Part model, mm, in its own coordinate system. Face numbers are marked on the shaded views. Round coordinates to 2 decimals unless told otherwise and drop trailing zeros. Loops run counter-clockwise (first coordinate to the right, second up) from the corner with the lowest first, then second, coordinate; pieces in that order, holes last.
from build123d import *

# Parameters (mm, degrees)
SKETCH1_W                   = 135
SKETCH1_H                   = 25
BOSS_EXTRUDE1_DEPTH         = 6
TAP_DRILL_FOR_M6X1_0_TAP1_D = 5
SKETCH2_R                   = 8
CUT_EXTRUDE1_DEPTH          = 70.688593041


with BuildPart() as part:
    # Sketch1 → Boss-Extrude1 (new, symmetric)
    with BuildSketch(Plane.XY):
        Rectangle(SKETCH1_W, SKETCH1_H)
    extrude(amount=BOSS_EXTRUDE1_DEPTH, both=True)

    # Tap Drill for M6x1.0 Tap1 (through all)
    with Locations(Plane.XY.offset(6)):
        with Locations((-22.5, 6), (-22.5, -6), (22.5, 6), (22.5, -6)):
            Hole(TAP_DRILL_FOR_M6X1_0_TAP1_D / 2)

    # Sketch2 → Cut-Extrude1 (cut, through all)
    with BuildSketch(Plane.XY.offset(6)):
        with Locations((-57.7, 0)):
            Circle(SKETCH2_R)
        with Locations((57.7, 0)):
            Circle(SKETCH2_R)
    extrude(amount=-CUT_EXTRUDE1_DEPTH, mode=Mode.SUBTRACT)


solid = part.part
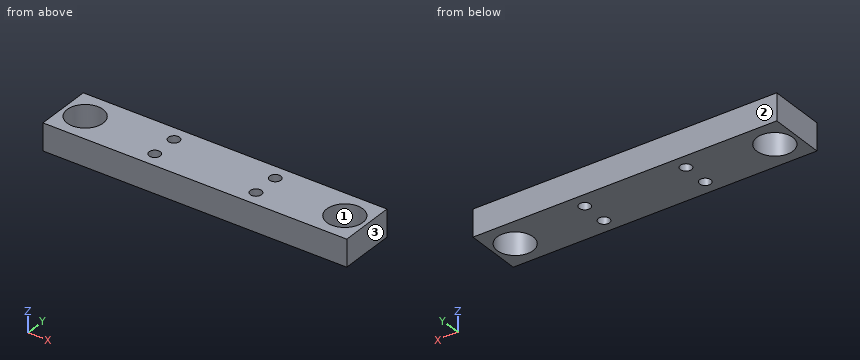
1) Wall check: line 1 along Y through (x, z) = (-22.5, 0); line 2 along X through (y, z) = (-0.5, -4.5); line 3 along Y through (x, z) = (-57.7, -0.5). Give the ranges that are in metal, low to high.
Values:
line 1: y = -12.5 to -8.5, -3.5 to 3.5, 8.5 to 12.5
line 2: x = -67.5 to -65.68, -49.72 to 49.72, 65.68 to 67.5
line 3: y = -12.5 to -8, 8 to 12.5
2) Slice it at A-A, the plane x = -57.7. Give the cut face in (y, z).
Values:
outline: (-12.5, -6) - (-8, -6) - (-8, 6) - (-12.5, 6) - close; (8, -6) - (12.5, -6) - (12.5, 6) - (8, 6) - close
3) Slice it at C-C, the plane x = -22.5. Give the cut face in (y, z), then the cut area to 3 significant figures.
Values:
outline: (-12.5, -6) - (-8.5, -6) - (-8.5, 6) - (-12.5, 6) - close; (-3.5, -6) - (3.5, -6) - (3.5, 6) - (-3.5, 6) - close; (8.5, -6) - (12.5, -6) - (12.5, 6) - (8.5, 6) - close
area: 180 mm2
4) Slice it at B-B, the plane z = -4.25. Give the cut face in (x, y).
Values:
outline: (-67.5, -12.5) - (67.5, -12.5) - (67.5, 12.5) - (-67.5, 12.5) - close; hole circle Ø16 at (-57.7, 0); hole circle Ø5 at (-22.5, -6); hole circle Ø5 at (-22.5, 6); hole circle Ø5 at (22.5, -6); hole circle Ø5 at (22.5, 6); hole circle Ø16 at (57.7, 0)
5) Slice it at D-D, the plane y = 6. Give the cut face in (x, z).
Values:
outline: (-67.5, -6) - (-62.99, -6) - (-62.99, 6) - (-67.5, 6) - close; (-52.41, -6) - (-25, -6) - (-25, 6) - (-52.41, 6) - close; (-20, -6) - (20, -6) - (20, 6) - (-20, 6) - close; (25, -6) - (52.41, -6) - (52.41, 6) - (25, 6) - close; (62.99, -6) - (67.5, -6) - (67.5, 6) - (62.99, 6) - close
6) Mould opens along X. For the marked faces 1, 2 and 3 say: released by +X, released by -X, zero draft, split by the parting line, or undercut.
Values:
face 1: undercut
face 2: zero draft
face 3: released by +X
